from build123d import *

# Parameters (mm, degrees)
IZIM1_R                     = 62
Y_KSEKLIK_EKSTR_ZYON1_DEPTH = 10
IZIM2_W                     = 60
IZIM2_H                     = 30
IZIM2_R                     = 1.5
IZIM2_W_2                   = 45
IZIM2_H_2                   = 15
Y_KSEKLIK_EKSTR_ZYON2_DEPTH = 25
DAIRESEL_KAPLAMA1_COUNT     = 2
DAIRESEL_KAPLAMA1_ANGLE     = 180
KES_EKSTR_ZYON1_START       = -3
IZIM4_W                     = 15
IZIM4_H                     = 40
KES_EKSTR_ZYON1_DEPTH       = 21
DAIRESEL_KAPLAMA2_COUNT     = 2
IZIM6_W                     = 4.288055231
IZIM6_H                     = 60
IZIM6_W_2                   = 1.841875029
KES_EKSTR_ZYON3_DEPTH       = 20
IZIM5_R                     = 40
KES_EKSTR_ZYON4_DEPTH       = 5
IZIM7_R                     = 5
KES_EKSTR_ZYON5_DEPTH       = 10


with BuildPart() as part:
    # Çizim1 → Yükseklik-Ekstrüzyon1 (new body)
    with BuildSketch(Plane.XY):
        Circle(IZIM1_R)
    extrude(amount=Y_KSEKLIK_EKSTR_ZYON1_DEPTH)

    # Çizim2 → Yükseklik-Ekstrüzyon2 (add)
    with BuildSketch(Plane(origin=(64, 0, 0), x_dir=(0, 0, -1), z_dir=(1, 0, 0))):
        with Locations((-30, 0)):
            Rectangle(IZIM2_W, IZIM2_H)
        with Locations((-5, 7.5)):
            Circle(IZIM2_R, mode=Mode.SUBTRACT)
        with Locations((-4.950442225, -7.5)):
            Circle(IZIM2_R, mode=Mode.SUBTRACT)
        with Locations((-32.5, 0)):
            Rectangle(IZIM2_W_2, IZIM2_H_2, mode=Mode.SUBTRACT)
    y_kseklik_ekstr_zyon2 = extrude(amount=-Y_KSEKLIK_EKSTR_ZYON2_DEPTH)

    # Dairesel Kaplama1: Yükseklik-Ekstrüzyon2 ×2 about axis
    dairesel_kaplama1_axis = Axis((-1.223090101, 0, 0), (0, 0, 1))
    for i in range(1, DAIRESEL_KAPLAMA1_COUNT):
        add(y_kseklik_ekstr_zyon2.rotate(dairesel_kaplama1_axis, i * DAIRESEL_KAPLAMA1_ANGLE / (DAIRESEL_KAPLAMA1_COUNT - 1)))

    # Çizim4 → Kes-Ekstrüzyon1 (cut)
    with BuildSketch(Plane.XZ.offset(-7.5).offset(KES_EKSTR_ZYON1_START)):
        with Locations((-53.946180202, 30)):
            Rectangle(IZIM4_W, IZIM4_H)
    kes_ekstr_zyon1 = extrude(amount=KES_EKSTR_ZYON1_DEPTH, mode=Mode.SUBTRACT)

    # Dairesel Kaplama2: Kes-Ekstrüzyon1 ×2 about axis
    dairesel_kaplama2_axis = Axis((-0.749102638, 0, 0), (0, 0, 1))
    for i in range(1, DAIRESEL_KAPLAMA2_COUNT):
        add(kes_ekstr_zyon1.rotate(dairesel_kaplama2_axis, i * 360 / DAIRESEL_KAPLAMA2_COUNT), mode=Mode.SUBTRACT)

    # Çizim6 → Kes-Ekstrüzyon3 (cut, symmetric)
    with BuildSketch(Plane(origin=(0, 0, 0), x_dir=(1, 0, 0), z_dir=(0, 1, 0))):
        with Locations((-64.302152587, -30)):
            Rectangle(IZIM6_W, IZIM6_H)
        with Locations((63.079062486, -30)):
            Rectangle(IZIM6_W_2, IZIM6_H)
    extrude(amount=KES_EKSTR_ZYON3_DEPTH, both=True, mode=Mode.SUBTRACT)

    # Çizim5 → Kes-Ekstrüzyon4 (cut)
    with BuildSketch(Plane.XY.offset(10)):
        with Locations((-1.443493492, 0.137209833)):
            Circle(IZIM5_R)
    extrude(amount=-KES_EKSTR_ZYON4_DEPTH, mode=Mode.SUBTRACT)

    # Çizim7 → Kes-Ekstrüzyon5 (cut)
    with BuildSketch(Plane(origin=(0, 0, 0), x_dir=(-1, 0, 0), z_dir=(0, 0, -1))):
        Circle(IZIM7_R)
    extrude(amount=-KES_EKSTR_ZYON5_DEPTH, mode=Mode.SUBTRACT)


solid = part.part
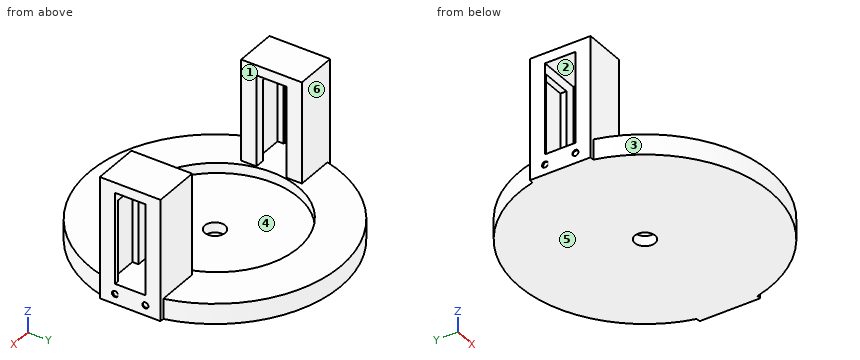
Design review of the part built by this model. Coordinates are the model's own, in mm. Face numbers are marked on the shaded views. A direction names the side the tool comes from. Round coordinates to 2 decimals unless told otherwise and drop trailing zeros. Write each loop counter-clockwise with the first axis right and the second up, starting at its lowest first coordinate (ties: lowest second). Pieces come first, ordered by that corner, then holes. Notation, with made-up numbers: (27, -33) - (61, -33) arc R19 cw to (61, -16) - close; hole circle Ø10 at (-21, 62). An arc over 180 degrees is marked (long way). Use a Markdown table: item, result. Add a question column.
1. We need section A-A (z = 37). Count the separate pieces of the cut face and the enclosed holes in it, then the cut area to 3 significant figures.
2. Wall thickness on probe 1 along Z at (x, y) = (61, -7); probe 2 along Y at (x, z) = (0, 3); probe 3 along Y at (x, z) = (-46, 23.5): over which ranges is each line inside the solid? List them lowest first.
3. For the marked faces 1, 2 and 3, list the 3-axis set-ups (+Z, -Z, +X, -X, +Y, -Y) from which the entire face can be reached by the end or side of a thin tool; tool diameter is ignored.
4. Clearance check with flat-ended pins moving along their axes: pin 1 (2.5 mm diameter, centred on y = -7.5, z = 5, fed in from +X); pin 2 (0.9 mm diameter, centred on x = 50, y = 9.5, fed in from -Z); pin 3 (7.5 mm diameter, centred on x = -53.5, z = 25, fed in from +Y); pin 4 (5 mm diameter, centred on x = 40.5, y = 42.5, fed in from +Z). State where each tip first meets the part, or that it passes through.
5. We need section B-B (x = -50.5). State the section outline as (y, z) points.
6. Mouldability with a two-part tool opening along Y and no side actions: class the marked faces 4, 5 and 6 as +Y half, -Y half, draft (parallel to the pull), parting line (faces both ways), or undercut.
7. We need section C-C (x = 0). State the section outline as (y, z) points, then the cut area to 3 significant figures.
8. We need section D-D (y = -19). State the section outline as (x, z) points, then the cut area to 3 significant figures.
Output:
| question | item | result |
|---|---|---|
| 1 | separate pieces | 4 |
| 1 | enclosed holes | 0 |
| 1 | area | 478 mm2 |
| 2 | probe 1 | z = 0 to 10, 55 to 60 |
| 2 | probe 2 | y = -62 to -5, 5 to 62 |
| 2 | probe 3 | y = -15 to -7.5, 7.5 to 15 |
| 3 | face 1 | +Z, +Y, -Y |
| 3 | face 2 | +X, -X |
| 3 | face 3 | +Z, -Z, -Y |
| 4 | pin 1 | stops at x = 61.68 |
| 4 | pin 2 | stops at z = 0 |
| 4 | pin 3 | stops at y = 15 |
| 4 | pin 4 | stops at z = 10 |
| 5 | outline | (-35.97, 0) - (35.97, 0) - (35.97, 10) - (15, 10) - (15, 60) - (-15, 60) - (-15, 10) - (-35.97, 10) - close; hole (-10.5, 10) - (10.5, 10) - (10.5, 50) - (7.5, 50) - (7.5, 55) - (-7.5, 55) - (-7.5, 50) - (-10.5, 50) - close |
| 6 | face 4 | undercut |
| 6 | face 5 | draft |
| 6 | face 6 | +Y half |
| 7 | outline | (-62, 0) - (-5, 0) - (-5, 5) - (-39.84, 5) - (-39.84, 10) - (-62, 10) - close; (5, 0) - (62, 0) - (62, 10) - (40.11, 10) - (40.11, 5) - (5, 5) - close |
| 7 | area | 790 mm2 |
| 8 | outline | (-59.02, 0) - (59.02, 0) - (59.02, 10) - (33.68, 10) - (33.68, 5) - (-36.57, 5) - (-36.57, 10) - (-59.02, 10) - close |
| 8 | area | 829 mm2 |
